from build123d import *

# Parameters (mm, degrees)
F0_W      = 209.55
F0_H      = 25.4
F1_DEPTH  = 101.6
F2_W      = 38.1
F2_H      = 38.1
F3_DEPTH  = 25.401
F5_DEPTH  = 25.4
F6_W      = 82.55
F6_H      = 101.6
F7_DEPTH  = 25.4
F9_DEPTH  = 76.2
F10_W     = 50.8
F10_H     = 25.4
F11_DEPTH = 50.8
F12_R     = 12.7


with BuildPart() as f1:
    # F0 (on Front) → F1 (new body)
    with BuildSketch(Plane.XZ):
        with Locations((104.775, 12.7)):
            Rectangle(F0_W, F0_H)
    extrude(amount=F1_DEPTH)

    # F2 (on face) → F3 (cut, through all)
    with BuildSketch(Plane.XY.offset(25.4)):
        with Locations((19.05, -50.8)):
            Rectangle(F2_W, F2_H)
        with Locations((190.5, -50.8)):
            Rectangle(F2_W, F2_H)
    extrude(amount=-F3_DEPTH, mode=Mode.SUBTRACT)

    # F4 (on face) → F5 (join)
    with BuildSketch(Plane(origin=(0, 0, 0), x_dir=(1, 0, 0), z_dir=(0, 0, -1))):
        Polygon((171.45, 101.6), (38.1, 101.6), (38.1, 69.85), (38.1, 31.75), (38.1, 0), (171.45, 0), (171.45, 31.75), (171.45, 69.85), align=None)
    extrude(amount=F5_DEPTH)

    # F6 (on face) → F7 (cut)
    with BuildSketch(Plane(origin=(0, 0, -25.4), x_dir=(1, 0, 0), z_dir=(0, 0, -1))):
        with Locations((104.775, 50.8)):
            Rectangle(F6_W, F6_H)
    extrude(amount=-F7_DEPTH, mode=Mode.SUBTRACT)

    # F8 (on face) → F9 (join)
    with BuildSketch(Plane.XY.offset(25.4)):
        Polygon((158.75, 0), (57.15, 0), (107.95, -101.6), align=None)
    extrude(amount=F9_DEPTH)

    # F10 (on face) → F11 (cut)
    with BuildSketch(Plane.XZ.offset(101.6)):
        with Locations((107.95, 63.5)):
            Rectangle(F10_W, F10_H)
    extrude(amount=-F11_DEPTH, mode=Mode.SUBTRACT)

    # F12
    f12_edges = [f1.edges().sort_by_distance(p)[0] for p in [
        (0, -101.6, 12.7),
        (0, -69.85, 12.7),
        (0, -31.75, 12.7),
        (0, 0, 12.7),
        (209.55, 0, 12.7),
        (209.55, -31.75, 12.7),
        (209.55, -69.85, 12.7),
        (209.55, -101.6, 12.7),
        (63.5, -50.8, 0),
        (146.05, -50.8, 0),
    ]]
    fillet(f12_edges, radius=F12_R)


solid = f1.part
Here's how the part is built. I have some questions about the finished solid (model axes, mm). A direction names the side the tool comes from. Coordinates: 2 decimals unless noted, no trailing zeros. Write each loop counter-clockwise with the first axis right and the second up, starting at its lowest first coordinate (ties: lowest second). Pieces come first, ordered by that corner, then holes.
Item 1: I want a section at D-D on y = -37.5. Write out the boundary of the cut face in (x, z).
Item 2: I want a section at A-A on y = -54. Write out the boundary of the cut face in (x, z).
Item 3: If I drill on line 1 (Y direction, x = 185, z = 6); line 2 (X direction, y = -37, z = -19.5); line 3 (Z direction, x = 43, y = -35.5), over which ranges is the centre line in solid material (lowest first)?
Item 4: If we mould it in two halves opening along Z, with no side actions, what happens to faces 1 (the flat face through (209.55, -86, 13)), 2 (the cylindrical face through (142.23, -51.51, -3.62)), 3 (the flat face through (108, -50.8, 64)), 4 (the flat face through (107, -39, 101.6))? For each: +Z half, -Z half, draft (parallel to the pull), parting line (faces both ways), or undercut.
Item 5: Will these pins go through, and if not, where does the flat tip stop? pin 1 (6.5 mm diameter, centred on y = -54.5, z = -17, fed in from -X); pin 2 (15 mm diameter, centred on x = 114.5, y = -83, fed in from -Z); pin 3 (6 mm diameter, centred on y = -26, z = 24.5, fed in from -X).
Item 6: On a 3-axis mill with a long thin cutter (end or side, diameter ignored), from which of +Z, -Z, +X, -X, +Y, -Y can I reach the whole of each face in a straight line? I mean faces 5 (the cylindrical face through (67.12, -51.51, -3.82)), 6 (the cylindrical face through (3.62, -73.67, 12.52)), 7 (the flat face through (190, -86, 0)). Say none if no direction works.
Item 7: I want a section at C-C on z = 12.5. Write out the boundary of the cut face in (x, y).
Item 8: I want a section at B-B on x = 177.5. Write out the boundary of the cut face in (y, z).
Findings below:
1. outline: (38.1, -25.4) - (63.5, -25.4) - (63.5, -12.7) arc R12.7 cw to (76.2, 0) - (133.35, 0) arc R12.7 cw to (146.05, -12.7) - (146.05, -25.4) - (171.45, -25.4) - (171.45, 25.4) - (140, 25.4) - (140, 101.6) - (75.9, 101.6) - (75.9, 25.4) - (38.1, 25.4) - close
2. outline: (38.1, -25.4) - (63.5, -25.4) - (63.5, -12.7) arc R12.7 cw to (76.2, 0) - (133.35, 0) arc R12.7 cw to (146.05, -12.7) - (146.05, -25.4) - (171.45, -25.4) - (171.45, 25.4) - (131.75, 25.4) - (131.75, 50.8) - (84.15, 50.8) - (84.15, 25.4) - (38.1, 25.4) - close; (84.15, 76.2) - (131.75, 76.2) - (131.75, 101.6) - (84.15, 101.6) - close
3. line 1: y = -101.6 to -69.85, -31.75 to 0
3. line 2: x = 38.1 to 63.5, 146.05 to 171.45
3. line 3: z = -25.4 to 25.4
4. face 1: draft
4. face 2: -Z half
4. face 3: undercut
4. face 4: +Z half
5. pin 1: stops at x = 38.1
5. pin 2: stops at z = 0
5. pin 3: stops at x = 0.63
6. face 5: -Z, +Y, -Y
6. face 6: +Z, -Z, -X
6. face 7: -Z, +X, +Y, -Y
7. outline: (0, -88.9) arc R12.7 ccw to (12.7, -101.6) - (196.85, -101.6) arc R12.7 ccw to (209.55, -88.9) - (209.55, -82.55) arc R12.7 ccw to (196.85, -69.85) - (171.45, -69.85) - (171.45, -31.75) - (196.85, -31.75) arc R12.7 ccw to (209.55, -19.05) - (209.55, -12.7) arc R12.7 ccw to (196.85, 0) - (12.7, 0) arc R12.7 ccw to (0, -12.7) - (0, -19.05) arc R12.7 ccw to (12.7, -31.75) - (38.1, -31.75) - (38.1, -69.85) - (12.7, -69.85) arc R12.7 ccw to (0, -82.55) - close
8. outline: (-101.6, 0) - (-69.85, 0) - (-69.85, 25.4) - (-101.6, 25.4) - close; (-31.75, 0) - (0, 0) - (0, 25.4) - (-31.75, 25.4) - close
